Input: part model. Units: mm. Frame: model coordinates. A direction names the side the tool comes from. Coordinates: 2 decimals unless noted, no trailing zeros. Write each loop counter-clockwise with the first axis right and the second up, starting at its lowest first coordinate (ties: lowest second). Pieces come first, ordered by that corner, then holes. Notation, with made-up numbers: (54, -26.5) - (99, -26.5) arc R26 ccw to (99, -4.5) - close; hole circle Ø7 at (-34.75, 32). An arc over 180 degrees is marked (long way). Use a Markdown table: item, result. Add a question column.
Q1. Section query C-C (y = 2.25). Return the cut outline in (x, z), then the cut area to 3 significant figures.
Q2. Set-up query: faces 1 (the face through (-5, -4, 0)), 2 (the face through (56.526, 2.028, -0.481)). Return all of +Z, -Z, +X, -X, +Y, -Y with unobstructed straight access to the full face (end or side cutting, diameter ignored); none if empty.
Q3. Pin query (flat end, axial travel): P1, Ø5, axis at x = 33.5, z = -1, coming from the -Y side; P2, Ø2, axis at y = -5.5, z = -0.5, coming from the +X side; P3, Ø1, axis at y = -8, z = -1.5, coming from the +X side. Return the tip coordinate at first contact, or that it passes through.
Q4. Material intervals for probe 1 along X at (y, z) = (2.8, 0); probe 2 along X at (y, z) = (3.25, -1.25); probe 3 along Z at (x, y) = (27.5, 3), sorted ascending. Write a range as from..to.
Q5. Section query A-A (z = 0). Return the cut outline in (x, y).
Q6. Section query D-D (z = 3). Return the cut outline in (x, y), then the cut area to 3 significant figures.
Q7. Section query B-B (x = 27.5). Return the cut outline in (y, z), then the cut area to 3 significant figures.
Q8. Mould query, pull axis X, two halves, no side actions, for faces 3 (the face through (60, 2, 0)), 4 (the face through (26.32, 2.03, -1.08)), 5 (the face through (28, 4, -2)). Classes: released by +X, released by -X, zero draft, split by the parting line, or undercut.
from build123d import *

# Parameters (mm, degrees)
BOSS_EXTRUDE1_DEPTH = 4
SKETCH3_R           = 5
BOSS_EXTRUDE2_DEPTH = 10
SKETCH2_R           = 1.6
CUT_EXTRUDE1_DEPTH  = 15


with BuildPart() as part:
    # Sketch1 → Boss-Extrude1 (new body)
    with BuildSketch(Plane(origin=(0, 0, 0), x_dir=(1, 0, 0), z_dir=(0, 1, 0))):
        with BuildLine():
            Line((0, 5), (55, 5))
            ThreePointArc((55, 5), (60, 0), (55, -5))
            Line((55, -5), (0, -5))
            ThreePointArc((0, -5), (-5, 0), (0, 5))
        make_face()
    extrude(amount=BOSS_EXTRUDE1_DEPTH)

    # Sketch3 → Boss-Extrude2 (add)
    with BuildSketch(Plane.XZ):
        Circle(SKETCH3_R)
    extrude(amount=BOSS_EXTRUDE2_DEPTH)

    # Sketch2 → Cut-Extrude1 (cut, through all)
    with BuildSketch(Plane(origin=(0, 4, 0), x_dir=(1, 0, 0), z_dir=(0, 1, 0))):
        Circle(SKETCH2_R)
        with Locations((27.5, 0)):
            Circle(SKETCH2_R)
        with Locations((55, 0)):
            Circle(SKETCH2_R)
    extrude(amount=-CUT_EXTRUDE1_DEPTH, mode=Mode.SUBTRACT)


solid = part.part
Values follow:
| question | item | result |
|---|---|---|
| 1 | outline | (0, -5) - (55, -5) arc R5 ccw to (55, 5) - (0, 5) arc R5 ccw to start; hole circle Ø3.2 at (0, 0); hole circle Ø3.2 at (27.5, 0); hole circle Ø3.2 at (55, 0) |
| 1 | area | 604 mm2 |
| 2 | face 1 | -Y |
| 2 | face 2 | +Y, -Y |
| 3 | P1 | y = 0 |
| 3 | P2 | x = 5 |
| 3 | P3 | x = 4.9 |
| 4 | probe 1 | -5..-1.6, 1.6..25.9, 29.1..53.4, 56.6..60 |
| 4 | probe 2 | -4.84..-1, 1..26.5, 28.5..54, 56..59.84 |
| 4 | probe 3 | -5..-1.6, 1.6..5 |
| 5 | outline | (-5, -10) - (-1.6, -10) - (-1.6, 4) - (-5, 4) - close; (1.6, -10) - (5, -10) - (5, 0) - (25.9, 0) - (25.9, 4) - (1.6, 4) - close; (29.1, 0) - (53.4, 0) - (53.4, 4) - (29.1, 4) - close; (56.6, 0) - (60, 0) - (60, 4) - (56.6, 4) - close |
| 6 | outline | (-4, -10) - (4, -10) - (4, 0) - (59, 0) - (59, 4) - (-4, 4) - close |
| 6 | area | 332 mm2 |
| 7 | outline | (0, -5) - (4, -5) - (4, -1.6) - (0, -1.6) - close; (0, 1.6) - (4, 1.6) - (4, 5) - (0, 5) - close |
| 7 | area | 27.2 mm2 |
| 8 | face 3 | released by +X |
| 8 | face 4 | undercut |
| 8 | face 5 | zero draft |
